Answer from the drawing. Dimensions are ordinates in mm from the lowest x, y and z of the part. Give positions to 0.01 mm unless a question says otherwise; leave off trailing zeros. Write each loop counter-clockwise with the first axis right and the second up, starting at its lowest first coordinate (ties: lowest second). Pieces come first, ordered by that corner, then holes.
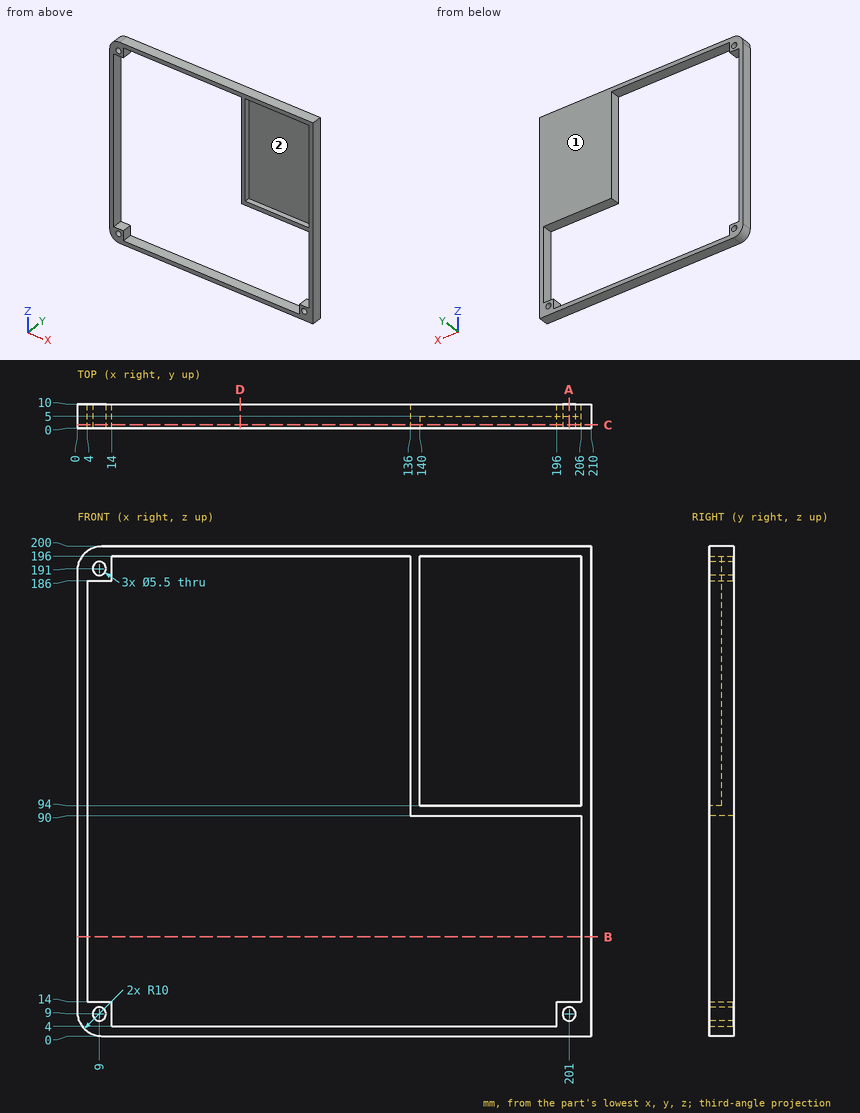
Item 1: Section C-C (y = 1.5) is taken. Write down the section's boundary in (x, z), and give its area (3 significant figures).
Result set:
outline: (0, 10) arc R10 ccw to (10, 0) - (210, 0) - (210, 200) - (10, 200) arc R10 ccw to (0, 190) - close; hole (4, 14) - (14, 14) - (14, 4) - (196, 4) - (196, 14) - (206, 14) - (206, 90) - (136, 90) - (136, 196) - (14, 196) - (14, 186) - (4, 186) - close; hole circle Ø5.5 at (9, 9); hole circle Ø5.5 at (9, 191); hole (140, 94) - (206, 94) - (206, 196) - (140, 196) - close; hole circle Ø5.5 at (201, 9)
area: 4,090 mm2
Item 2: Section B-B (z = 40.5) is taken. Write down the section's boundary in (x, y), and give its area (3 significant figures).
Result set:
outline: (0, 0) - (4, 0) - (4, 10) - (0, 10) - close; (206, 0) - (210, 0) - (210, 10) - (206, 10) - close
area: 80.0 mm2
Item 3: Find the intervals of material crossed by line 1 along X through (y, z) = (6.5, 191); line 2 along X through (y, z) = (6.25, 9); line 3 along Z through (x, y) = (145, 4.5), in increasing order.
Result set:
line 1: x = 0.05 to 6.25, 11.75 to 14, 136 to 210
line 2: x = 0.05 to 6.25, 11.75 to 14, 196 to 198.25, 203.75 to 210
line 3: z = 0 to 4, 90 to 94, 196 to 200
Item 4: Section A-A (x = 201) is taken. Write down the section's boundary in (y, z), and give its area (3 significant figures).
Result set:
outline: (0, 0) - (10, 0) - (10, 6.25) - (0, 6.25) - close; (0, 11.75) - (10, 11.75) - (10, 14) - (0, 14) - close; (0, 90) - (10, 90) - (10, 200) - (0, 200) - (0, 196) - (5, 196) - (5, 94) - (0, 94) - close
area: 675 mm2
Item 5: Determine the mould class of the marked faces 1 and 2 for opening direction Z: pulls with the +Z half, pulls with the -Z half, needs draft (parallel to the pull), parting line crosses it, or undercut.
Result set:
face 1: needs draft
face 2: undercut
Item 6: Section D-D (x = 66.5) is taken. Write down the section's boundary in (y, z).
Result set:
outline: (0, 0) - (10, 0) - (10, 4) - (0, 4) - close; (0, 196) - (10, 196) - (10, 200) - (0, 200) - close
Item 7: This flat-tipped pin is pushed along its axis until it touches: pin 1 Ø20 at (x, z) = (177, 127.5) entering from -Y. Where does it stop, or does it pass through?
Result set:
pin 1: stops at y = 5
